Part model, mm, in its own coordinate system. Face numbers are marked on the shaded views. A direction names the side the tool comes from. Coordinates: 2 decimals unless noted, no trailing zeros. Write each loop counter-clockwise with the first axis right and the second up, starting at its lowest first coordinate (ties: lowest second). Pieces come first, ordered by that corner, then holes. Notation, with made-up numbers: (11.25, 60) -> (61.25, 60) arc R24 ccw to (61.25, 99) -> close; hole circle Ø4 at (1, -16.75). An arc over 180 degrees is marked (long way). Write item = value, one per line. Start each with the question number.
Q1. Pull direction Z, two halves, no side cores. Call the marked faces 1, 2 and 3: released by +Z, released by -Z, zero draft, split by the parting line, or undercut.
Q2. Band-saw the part on B-B, the plane z = 0. List the corners of the cut face in (x, y).
Q3. Band-saw the part on A-A, the plane x = 0. List the corners of the cut face in (y, z).
Q4. Pin check, flat tips, straight feed: P1, Ø7, axis at x = 0, z = 20, coming from the +Y side; P2, Ø2, axis at y = 27.5, z = 26.5, coming from the -X side; P3, Ø1, axis at x = -36, z = 15, coming from the -Y side; P4, Ø2, axis at x = -21, y = 34, coming from the -Z side. Stop position of each tip, or through.
Q5. Probe line 1 (Y direction, x = 55, z = -8.5); line 2 (Y direction, x = 19.5, z = 9); line 3 (X direction, y = 28.5, z = -10). List the from-to ranges inside material, lowest first.
Q6. Tool access for the marked faces 4 and 5: list every direction of +Z, -Z, +X, -X, +Y, -Y with a clear straight run to the whole face (end or side of a thin tool).
from build123d import *

# Parameters (mm, degrees)
M6X0_5_TAPPED_HOLE1_D = 5.5
CIRPATTERN1_COUNT     = 3
CHAMFER1_SIZE         = 3
SKETCH7_R             = 5
CUT_EXTRUDE1_DEPTH    = 5


with BuildPart() as part:
    # Sketch1 → Revolve1 (revolve)
    with BuildSketch(Plane(origin=(0, 0, 0), x_dir=(0, 0, -1), z_dir=(1, 0, 0))):
        Polygon((0, 0), (-78, 0), (-78, 20), (-55, 20), (-55, 40), (-30, 40), (-30, 35), (0, 35), align=None)
    revolve(axis=Axis((0, 226.154402008, 0), (0, -1, 0)))

    # M6x0.5 Tapped Hole1 (through all)
    with Locations(Plane(origin=(0, 0, 20), x_dir=(0, 0, -1), z_dir=(0, -1, 0))):
        with Locations((0, 0)):
            m6x0_5_tapped_hole1 = Hole(M6X0_5_TAPPED_HOLE1_D / 2)

    # CirPattern1: M6x0.5 Tapped Hole1 ×3 about axis
    cirpattern1_axis = Axis((0, 0, 0), (0, 1, 0))
    for i in range(1, CIRPATTERN1_COUNT):
        add(m6x0_5_tapped_hole1.rotate(cirpattern1_axis, i * 360 / CIRPATTERN1_COUNT), mode=Mode.SUBTRACT)

    # Chamfer1
    chamfer1_edges = [part.edges().sort_by_distance(p)[0] for p in [
        (0, 40, -55),
        (0, 20, -78),
        (0, 0, -78),
    ]]
    chamfer(chamfer1_edges, length=CHAMFER1_SIZE)

    # Sketch7 → Cut-Extrude1 (cut)
    with BuildSketch(Plane.XZ):
        with Locations(Location((0, 20, 0), (0, 0, 270))):
            Circle(SKETCH7_R)
        with Locations(Location((17.320508076, -10, 0), (0, 0, 270))):
            Circle(SKETCH7_R)
        with Locations(Location((-17.320508076, -10, 0), (0, 0, 270))):
            Circle(SKETCH7_R)
    extrude(amount=-CUT_EXTRUDE1_DEPTH, mode=Mode.SUBTRACT)


solid = part.part
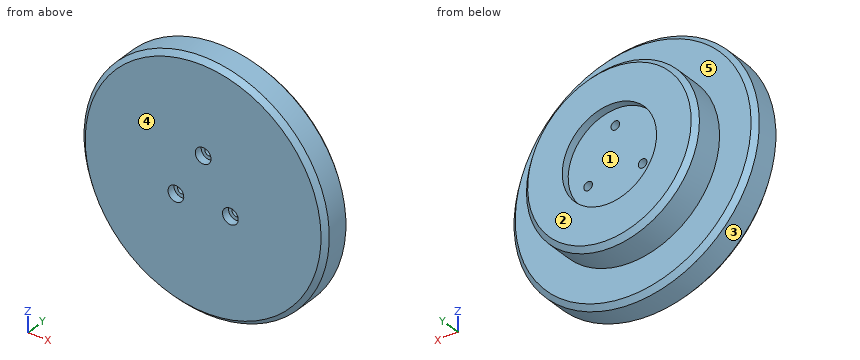
Ans:
q1.face_1 = undercut
q1.face_2 = zero draft
q1.face_3 = split by the parting line
q2.outline = (-78, 3) -> (-75, 0) -> (75, 0) -> (78, 3) -> (78, 17) -> (75, 20) -> (55, 20) -> (55, 37) -> (52, 40) -> (30, 40) -> (30, 35) -> (-30, 35) -> (-30, 40) -> (-52, 40) -> (-55, 37) -> (-55, 20) -> (-75, 20) -> (-78, 17) -> close
q3.outline = (0, -75) -> (3, -78) -> (17, -78) -> (20, -75) -> (20, -55) -> (37, -55) -> (40, -52) -> (40, -30) -> (35, -30) -> (35, 17.25) -> (5, 17.25) -> (5, 15) -> (0, 15) -> close; (0, 25) -> (5, 25) -> (5, 22.75) -> (35, 22.75) -> (35, 30) -> (40, 30) -> (40, 52) -> (37, 55) -> (20, 55) -> (20, 75) -> (17, 78) -> (3, 78) -> (0, 75) -> close
q4.P1 = 35
q4.P2 = -48.73
q4.P3 = 0
q4.P4 = -51.23
q5.line_1 = 0 to 20
q5.line_2 = 0 to 35
q5.line_3 = -54.08 to -20.07, -14.57 to 14.57, 20.07 to 54.08
q6.face_4 = +Z, -Z, +X, -X, -Y
q6.face_5 = +Y
